Input: part model. Units: mm. Frame: model coordinates. A direction names the side the tool comes from. Give positions to 0.01 mm unless a question says otherwise; leave off trailing zeros. Write each loop counter-clockwise with the first axis right and the second up, starting at its lowest first coordinate (ties: lowest second). Pieces come first, ordered by that corner, then holes.
```python
from build123d import *

# Parameters (mm, degrees)
SKETCH1_W               = 35
SKETCH1_H               = 20
BOSS_EXTRUDE1_DEPTH     = 40
SKETCH2_W               = 15
SKETCH2_H               = 20
BOSS_EXTRUDE2_DEPTH     = 16
SKETCH3_R               = 5
CUT_EXTRUDE1_DEPTH      = 26
FILLET3_R               = 3
SKETCH4_W               = 32
SKETCH4_H               = 34
CUT_EXTRUDE2_DEPTH      = 21
SKETCH5_R               = 2.5
CUT_EXTRUDE3_DEPTH      = 36
SKETCH7_W               = 10
SKETCH7_H               = 5
CUT_EXTRUDE4_DEPTH      = 21
FILLET5_R               = 2
SKETCH8_W               = 20
SKETCH8_H               = 4.66822317
CUT_EXTRUDE5_DEPTH      = 18.5
CUT_EXTRUDE5_DEPTH_BACK = 18.5


with BuildPart() as part:
    # Sketch1 → Boss-Extrude1 (new body)
    with BuildSketch(Plane(origin=(0, 0, 0), x_dir=(1, 0, 0), z_dir=(0, 1, 0))):
        with Locations((0, 10)):
            Rectangle(SKETCH1_W, SKETCH1_H)
    extrude(amount=BOSS_EXTRUDE1_DEPTH)

    # Sketch2 → Boss-Extrude2 (add)
    with BuildSketch(Plane.XZ):
        with Locations((0, -10)):
            Rectangle(SKETCH2_W, SKETCH2_H)
    extrude(amount=BOSS_EXTRUDE2_DEPTH)

    # Sketch3 → Cut-Extrude1 (cut, through all)
    with BuildSketch(Plane.ZY.offset(7.5)):
        with Locations((-10, -6)):
            Circle(SKETCH3_R)
    extrude(amount=-CUT_EXTRUDE1_DEPTH, mode=Mode.SUBTRACT)

    # Fillet3
    fillet3_edges = [part.edges().sort_by_distance(p)[0] for p in [
        (7.5, -16, -10),
        (-7.5, -16, -10),
    ]]
    fillet(fillet3_edges, radius=FILLET3_R)

    # Sketch4 → Cut-Extrude2 (cut, through all)
    with BuildSketch(Plane.XY):
        with Locations((0, 23)):
            Rectangle(SKETCH4_W, SKETCH4_H)
    extrude(amount=-CUT_EXTRUDE2_DEPTH, mode=Mode.SUBTRACT)

    # Sketch5 → Cut-Extrude3 (cut, through all)
    with BuildSketch(Plane.ZY.offset(17.5)):
        with Locations((-10, 37)):
            Circle(SKETCH5_R)
    extrude(amount=-CUT_EXTRUDE3_DEPTH, mode=Mode.SUBTRACT)

    # Sketch7 → Cut-Extrude4 (cut, through all)
    with BuildSketch(Plane(origin=(0, 0, -20), x_dir=(-1, 0, 0), z_dir=(0, 0, -1))):
        with Locations((12.5, 2.5)):
            Rectangle(SKETCH7_W, SKETCH7_H)
        with Locations((-12.5, 2.5)):
            Rectangle(SKETCH7_W, SKETCH7_H)
    extrude(amount=-CUT_EXTRUDE4_DEPTH, mode=Mode.SUBTRACT)

    # Fillet5
    fillet5_edges = [part.edges().sort_by_distance(p)[0] for p in [
        (7.5, 5, -10),
        (-7.5, 5, -10),
    ]]
    fillet(fillet5_edges, radius=FILLET5_R)

    # Sketch8 → Cut-Extrude5 (cut, two sides)
    with BuildSketch(Plane(origin=(0, 0, 0), x_dir=(0, 0, -1), z_dir=(1, 0, 0))) as cut_extrude5_sk:
        with Locations((10, -13.665888415)):
            Rectangle(SKETCH8_W, SKETCH8_H)
    extrude(amount=CUT_EXTRUDE5_DEPTH, mode=Mode.SUBTRACT)
    extrude(cut_extrude5_sk.sketch, amount=-CUT_EXTRUDE5_DEPTH_BACK, mode=Mode.SUBTRACT)


solid = part.part
```
Q1. Section A-A, the plane y = 37. Return the cut outline in (x, z), then the cut area to 3 significant figures.
Q2. Section B-B, the plane z = -10. Return the cut outline in (x, y), then the cut area to 3 significant figures.
Q3. Pin query (flat end, axial travel): pin 1 (6 mm diameter, centred on y = -6, z = -10, fed in from +X); pin 2 (4 mm diameter, centred on y = 1, z = -6, fed in from +X); pin 3 (6.5 mm diameter, centred on y = 37, z = -10, fed in from -X); pin 4 (4.5 mm diameter, centred on y = -7, z = -6.5, fed in from -X). Return the tip coordinate at first contact, or that it passes through.
Q4. Section C-C, the plane y = -6. Return the cut outline in (x, z).
Q5. Mould query, pull axis Y, two halves, no side actions, for faces 1 (the flat face through (17.5, 22, -10)), 2 (the flat face through (-13, 5, -10)), 3 (the flat face through (-17, 40, -10)), 4 (the cylindrical face through (16.74, 34.56, -10.54)). Classes: +Y half, -Y half, draft (parallel to the pull), parting line (faces both ways), or undercut.
Q6. Section D-D, the plane z = -6. Return the cut outline in (x, y).
Q7. Material intervals for line 1 along X through (y, z) = (7, -12.75); line 2 along Y through (x, z) = (-16.85, -10); line 3 along Y through (x, z) = (0.75, -10), sorted ascending.
Q8. Access query for faces 5 (the flat face through (-7.5, -1, -12)), 6 (the cylindrical face through (-16.76, 34.56, -10.54)), 7 (the flat face through (16, 23, -10)), 8 (the flat face through (14, 5, -10)). Directions: +Z, -Z, +X, -X, +Y, -Y. A direction counts if a zero-diameter tool reaches every point of the face in a straight line with its end or side. Return the directions, or none.
Solutions:
1. outline: (-17.5, -20) - (-16, -20) - (-16, -12.5) - (-17.5, -12.5) - close; (-17.5, -7.5) - (-16, -7.5) - (-16, 0) - (-17.5, 0) - close; (16, -20) - (17.5, -20) - (17.5, -12.5) - (16, -12.5) - close; (16, -7.5) - (17.5, -7.5) - (17.5, 0) - (16, 0) - close
1. area: 45.0 mm2
2. outline: (-17.5, 5) - (-9.5, 5) arc R2 cw to (-7.5, 3) - (-7.5, -1) - (7.5, -1) - (7.5, 3) arc R2 cw to (9.5, 5) - (17.5, 5) - (17.5, 34.5) - (16, 34.5) - (16, 6) - (-16, 6) - (-16, 34.5) - (-17.5, 34.5) - close; (-17.5, 39.5) - (-16, 39.5) - (-16, 40) - (-17.5, 40) - close; (-7.5, -11.33) - (7.5, -11.33) - (7.5, -11) - (-7.5, -11) - close; (16, 39.5) - (17.5, 39.5) - (17.5, 40) - (16, 40) - close
2. area: 219 mm2
3. pin 1: passes through
3. pin 2: stops at x = 7.5
3. pin 3: stops at x = -17.5
3. pin 4: stops at x = -7.5
4. outline: (-7.5, -20) - (7.5, -20) - (7.5, -15) - (-7.5, -15) - close; (-7.5, -5) - (7.5, -5) - (7.5, 0) - (-7.5, 0) - close
5. face 1: draft
5. face 2: -Y half
5. face 3: +Y half
5. face 4: undercut
6. outline: (-17.5, 5) - (-9.5, 5) arc R2 cw to (-7.5, 3) - (-7.5, -3) - (7.5, -3) - (7.5, 3) arc R2 cw to (9.5, 5) - (17.5, 5) - (17.5, 40) - (16, 40) - (16, 6) - (-16, 6) - (-16, 40) - (-17.5, 40) - close; (-7.5, -11.33) - (7.5, -11.33) - (7.5, -9) - (-7.5, -9) - close
7. line 1: x = -17.5 to -16, 16 to 17.5
7. line 2: y = 5 to 34.5, 39.5 to 40
7. line 3: y = -11.33 to -11, -1 to 6
8. face 5: +Z, -Z, -X, -Y
8. face 6: +X, -X
8. face 7: +Z, -Z, +Y
8. face 8: +Z, -Z, +X, -Y
